Source: CAD feature listing. Evaluate the final solid. Frame: model axes, mm. Face numbers are marked on the shaded views. A direction names the side the tool comes from. Coordinates: 2 decimals unless noted, no trailing zeros. Loops run counter-clockwise (first coordinate to the right, second up) from the corner with the lowest first, then second, coordinate; pieces in that order, holes last.
Item 1: Section query C-C, the plane z = 3.75. Return the cut outline in (x, y), then the cut area to 3 significant figures.
Item 2: Section query D-D, the plane y = 24. Return the cut outline in (x, z).
Item 3: Section query B-B, the plane x = 15. Return the cut outline in (y, z).
Item 4: Pin query (flat end, axial travel): pin 1 Ø5 at (x, y) = (15.5, -1.5) entering from -Z. Return the tip coordinate at first contact, or that it passes through.
Item 5: Section query A-A, the plane y = 10.5. Return the cut outline in (x, z), then the cut area to 3 significant figures.
Item 6: Line query: probe 1 along Y at (x, z) = (-4, 6.5); probe 2 along Y at (x, z) = (26, 7.75); probe 3 along X at (y, z) = (12.5, 5.75). Output: solid intervals per line, ascending.
Item 7: Pull-direction query (X, two-part tool) for the marked faces 1, 2, 3 and 4; classes: +X half, -X half, draft (parallel to the pull), parting line (faces both ways), or undercut.
Item 8: Reachability of the marked faces 5 and 6 from +Z, -Z, +X, -X, +Y, -Y: full face, straight path, thin tool, end or side. Return the list, or none.
Autodesk Inventor part; units mm, degrees
ref_plane "YZ Plane" through (0, 0, 0) normal (1, 0, 0) x (0, 1, 0)
ref_plane "XZ Plane" through (0, 0, 0) normal (0, 1, 0) x (-1, 0, 0)
ref_plane "XY Plane" through (0, 0, 0) normal (0, 0, 1) x (1, 0, 0)
sketch "Sketch1" plane through (0, 0, 0) normal (0, 0, 1) x (1, 0, 0)
  line L0 (0, 0) -> (22, 0)
  line L1 (22, 0) -> (22, 42)
  line L2 (22, 42) -> (0, 42)
  line L3 (0, 42) -> (0, 0)
  line L4 (-8, 50) -> (30, 50)
  line L5 (30, 50) -> (30, -8)
  line L6 (30, -8) -> (-8, -8)
  line L7 (-8, -8) -> (-8, 50)
  line L8 (0, 21) -> (22, 21) construction
  line L9 (11, 0) -> (11, 42) construction
  circle A0 centre (26, 10.5) radius 1.75
  circle A1 centre (26, 31.5) radius 1.75
  circle A2 centre (-4, 10.5) radius 1.75
  circle A3 centre (-4, 31.5) radius 1.75
  line L10 (0, 50) -> (22, 50)
  line L11 (22, 42) -> (0, 42)
  line L12 (0, 0) -> (22, 0)
  line L13 (22, -8) -> (0, -8)
  line L14 (5.4779, 42) -> (18.0265, 42)
  line L15 (5.4779, 0) -> (19.7232, 0)
  line L16 (0, 42) -> (0, 50)
  line L17 (22, 42) -> (22, 50)
  line L18 (0, 0) -> (0, -8)
  line L19 (22, 0) -> (22, -8)
  line L20 (-8, 50) -> (30, 50)
  line L21 (30, 50) -> (30, 53)
  line L22 (30, 53) -> (-8, 53)
  line L23 (-8, 53) -> (-8, 50)
  line L24 (-8, -8) -> (30, -8)
  line L25 (30, -8) -> (30, -11)
  line L26 (30, -11) -> (-8, -11)
  line L27 (-8, -11) -> (-8, -8)
  dimension "d0" = 42
  dimension "d2" = 8
  dimension "d3" = 3.5
  dimension "d4" = 10.5
  dimension "d5" = 4
  dimension "d6" = 8
  dimension "d15" = 22
  dimension "d16" = 22
  dimension "d17" = 22
  dimension "d18" = 3
  dimension "d19" = 38
  dimension "d20" = 38
  dimension "d21" = 3
extrude "Extrusion1" add sketch "Sketch1" along normal blind 10 contours L18 L6 L7 L4 L16 L3 | L0 L19 L6 L18 | L16 L4 L17 L2 | L6 L25 L26 L27 | L4 L23 L22 L21 | L19 L1 L17 L4 L5 L6
extrude "Extrusion2" cut sketch "Sketch1" along normal blind 6 contours L0 L19 L6 L18 | L16 L4 L17 L2
fillet "Fillet1" radius 8 2 edges at (30, -11, 5) (30, 53, 5)
fillet "Fillet2" radius 2 4 edges at (0, 42, 8) (0, 0, 8) (22, 0, 8) (22, 42, 8)
fillet "Fillet3" radius 2 12 edges at (27.6569, 50.6569, 10) (27.6569, -8.6569, 10) (7, -11, 10) (7, 53, 10) (27.6569, 50.6569, 0) (27.6569, -8.6569, 0) (7, -11, 0) (7, 53, 0) (11, 0, 10) (0, 21, 10) (11, 42, 10) (22, 21, 10)
equation "\"d0\" = MOUNT_LENGTH"
equation "\"d2\" = MOUNT_THICKNESS"
equation "\"d3\" = ThroughDiameter"
equation "\"d4\" = 0.25 * MOUNT_LENGTH"
equation "\"d5\" = 0.5 * MOUNT_THICKNESS"
equation "\"d15\" = MOUNT_WIDTH"
equation "\"d18\" = -0.5 * MOUNT_LENGTH + 0.5 * COXA_JOINT_LENGTH"
equation "\"d19\" = MOUNT_WIDTH + 2 * MOUNT_THICKNESS"
equation "\"d20\" = MOUNT_WIDTH + 2 * MOUNT_THICKNESS"
equation "\"d21\" = -0.5 * MOUNT_LENGTH + 0.5 * COXA_JOINT_LENGTH"
equation "\"d22\" = OUTER_FILLET"
equation "\"d13\" = INNER_FILLET"
equation "\"d23\" = INNER_FILLET"
equation "\"ThroughDiameter\" = 3.5"
properties part number "CoxaLeft"
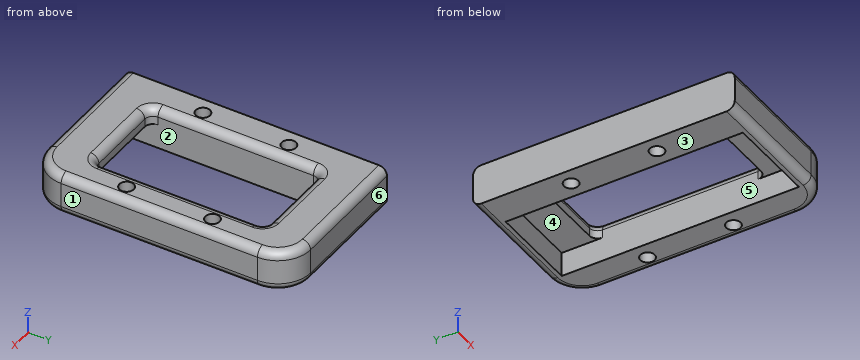
Verdict:
1. outline: (-8, -11) - (22, -11) arc R8 ccw to (30, -3) - (30, 45) arc R8 ccw to (22, 53) - (-8, 53) - close; hole circle Ø3.5 at (-4, 10.5); hole circle Ø3.5 at (-4, 31.5); hole (0, -8) - (22, -8) - (22, 50) - (0, 50) - close; hole circle Ø3.5 at (26, 10.5); hole circle Ø3.5 at (26, 31.5)
1. area: 1,090 mm2
2. outline: (-8, 0) - (0, 0) - (0, 8) arc R2 ccw to (-2, 10) - (-8, 10) - close; (22, 0) - (28, 0) arc R2 ccw to (30, 2) - (30, 8) arc R2 ccw to (28, 10) - (24, 10) arc R2 ccw to (22, 8) - close
3. outline: (-11, 2) arc R2 ccw to (-9, 0) - (-8, 0) - (-8, 6) - (0, 6) - (0, 8) arc R2 ccw to (-2, 10) - (-9, 10) arc R2 ccw to (-11, 8) - close; (42, 6) - (50, 6) - (50, 0) - (51, 0) arc R2 ccw to (53, 2) - (53, 8) arc R2 ccw to (51, 10) - (44, 10) arc R2 ccw to (42, 8) - close
4. pin 1: stops at z = 6
5. outline: (-8, 0) - (-5.75, 0) - (-5.75, 10) - (-8, 10) - close; (-2.25, 0) - (0, 0) - (0, 8) arc R2 ccw to (-2, 10) - (-2.25, 10) - close; (22, 0) - (24.25, 0) - (24.25, 10) - (24, 10) arc R2 ccw to (22, 8) - close; (27.75, 0) - (28, 0) arc R2 ccw to (30, 2) - (30, 8) arc R2 ccw to (28, 10) - (27.75, 10) - close
5. area: 86.6 mm2
6. probe 1: y = -11 to 8.75, 12.25 to 29.75, 33.25 to 53
6. probe 2: y = -9.93 to 8.75, 12.25 to 29.75, 33.25 to 51.93
6. probe 3: x = -8 to 0, 22 to 30
7. face 1: +X half
7. face 2: undercut
7. face 3: draft
7. face 4: undercut
8. face 5: -Z
8. face 6: +Z, -Z, +X, -X, +Y
